Geometry check sheet. Reference: the model listing, model coordinates, mm. A direction names the side the tool comes from. Give positions to 0.01 mm unless a question says otherwise; leave off trailing zeros. Loops run counter-clockwise (first coordinate to the right, second up) from the corner with the lowest first, then second, coordinate; pieces in that order, holes last. Notation, with made-up numbers: (69, 62.5) -> (92, 62.5) arc R18 cw to (92, 83.5) -> close; hole circle Ø5 at (-32.5, 46). An arc over 180 degrees is marked (long way). Answer as a JSON object with one key per item and string values.
Autodesk Inventor part; units mm, degrees
ref_plane "YZ Plane" through (0, 0, 0) normal (1, 0, 0) x (0, 1, 0)
ref_plane "XZ Plane" through (0, 0, 0) normal (0, 1, 0) x (-1, 0, 0)
ref_plane "XY Plane" through (0, 0, 0) normal (0, 0, 1) x (1, 0, 0)
sketch "Sketch1" plane through (0, 0, 0) normal (0, 0, 1) x (1, 0, 0)
  line L0 (64, 0) -> (64, 36)
  line L1 (64, 36) -> (0, 36)
  line L2 (0, 36) -> (0, 0)
  line L3 (40, 0) -> (40, -9)
  line L4 (40, -9) -> (24, -9)
  line L5 (24, -9) -> (24, 0)
  line L6 (0, 0) -> (24, 0)
  line L7 (40, 0) -> (64, 0)
  dimension "d0" = 64
  dimension "d1" = 36
  dimension "d2" = 16
  dimension "d3" = 9
  dimension "d4" = 24
extrude "Extrusion1" add sketch "Sketch1" along normal blind 32
sketch "Sketch2" plane through (0, 0, 32) normal (0, 0, 1) x (1, 0, 0)
  circle A0 centre (32, 20) radius 6
  line L0 (0, 36) -> (0, 0)
  line L1 (40, 0) -> (64, 0)
  arc A1 (45.5949, 28.4368) -> (18.4051, 28.4368) centre (32, 20) ccw
  line L2 (0, 8.4474) -> (4.331, 8.4474)
  line L3 (6.8801, 9.8655) -> (18.4051, 28.4368)
  line L4 (64, 0) -> (64, 36)
  line L5 (64, 8.4474) -> (59.669, 8.4474)
  line L6 (57.1199, 9.8655) -> (45.5949, 28.4368)
  arc A2 (4.331, 8.4474) -> (6.8801, 9.8655) centre (4.331, 11.4474) ccw
  arc A3 (57.1199, 9.8655) -> (59.669, 8.4474) centre (59.669, 11.4474) ccw
  line L7 (0, 8.4474) -> (0, 36)
  line L8 (64, 36) -> (0, 36)
  line L9 (0, 36) -> (64, 36)
  line L10 (64, 36) -> (64, 8.4474)
  point P0 (6, 8.4474)
  point P1 (58, 8.4474)
  point P2 (32, 36)
  dimension "d7" = 12
  dimension "d8" = 32
  dimension "d9" = 20
  dimension "d10" = 6
  dimension "d11" = 32
  dimension "d12" = 6
  dimension "d13" = 3
extrude "Extrusion2" cut sketch "Sketch2" against normal blind 22 contours L8 A1 L3 A2 L2 L0 | L8 L4 L5 A3 L6 A1
sketch "Sketch3" plane through (0, 0, 32) normal (0, 0, 1) x (1, 0, 0)
  circle A0 centre (32, 20) radius 8
  line L0 (0, 8.4474) -> (0, 36)
  line L1 (40, 0) -> (64, 0)
  point P0 (0, 0)
  dimension "d16" = 16
  dimension "d17" = 32
  dimension "d18" = 20
extrude "Extrusion3" cut sketch "Sketch3" against normal blind 24
sketch "Sketch4" plane through (0, 36, 0) normal (0, 1, 0) x (1, 0, 0)
  circle A0 centre (32, -20) radius 3
  line L0 (18.4051, -32) -> (45.5949, -32)
  line L1 (0, -32) -> (0, -10)
  point P0 (0, 0)
  dimension "d21" = 6
  dimension "d22" = 12
  dimension "d23" = 32
extrude "Extrusion4" cut sketch "Sketch4" against normal blind 16
sketch "Sketch5" plane through (0, 36, 0) normal (0, 1, 0) x (1, 0, 0)
  circle A0 centre (32, -20) radius 5
  line L0 (18.4051, -32) -> (45.5949, -32)
  line L1 (0, -32) -> (0, -10)
  point P0 (0, 0)
  dimension "d26" = 10
  dimension "d27" = 12
  dimension "d28" = 32
extrude "Extrusion5" cut sketch "Sketch5" against normal blind 4
sketch "Sketch6" plane through (24, -9, 0) normal (0, -1, 0) x (1, 0, 0)
  circle A0 centre (8, 24) radius 3
  circle A1 centre (8, 8) radius 3
  line L0 (0, 32) -> (16, 32)
  point P0 (-24, 0)
  dimension "d31" = 6
  dimension "d32" = 6
  dimension "d33" = 8
  dimension "d34" = 16
extrude "Extrusion6" cut sketch "Sketch6" against normal blind 16
properties part number "third"
1) Section check A-A on z = 30. Record the cut outline in (x, y).
Geometry check:
{"outline": "(0, 0) -> (24, 0) -> (24, -9) -> (40, -9) -> (40, 0) -> (64, 0) -> (64, 8.45) -> (59.67, 8.45) arc R3 cw to (57.12, 9.87) -> (45.59, 28.44) arc R16 ccw to (18.41, 28.44) -> (6.88, 9.87) arc R3 cw to (4.33, 8.45) -> (0, 8.45) -> close; hole circle Ø16 at (32, 20)"}
2) Section check C-C on y = -5. Record the cut outline in (x, z).
Geometry check:
{"outline": "(24, 0) -> (40, 0) -> (40, 32) -> (24, 32) -> close; hole circle Ø6 at (32, 8); hole circle Ø6 at (32, 24)"}
3) Tool access check on faces 5 (the face through (28, 34, 23)), 6 (the face through (55, 25, 10)), 7 (the face through (12, 0, 16)), 8 (the face through (2, 8.447, 21)). Record the directions out of +Z, -Z, +X, -X, +Y, -Y that give a thin tool (end or side, any length) a straight path to the whole face; none if there is none.
Geometry check:
{"face 5": "+Y", "face 6": "+Z, +X, +Y", "face 7": "+Z, -Z, -X, -Y", "face 8": "+Z, -X, +Y"}
4) Depth check by flat-ended pin: P1, Ø5, axis at x = 62.5, z = 25.5, coming from the +Y side; P2, Ø6, axis at x = 15.5, z = 27.5, coming from the +Y side; P3, Ø3, axis at x = 30.5, z = 19, coming from the +Y side. Enter the tip coordinate at first touch or a pass-through.
Geometry check:
{"P1": "stops at y = 8.45", "P2": "stops at y = 28.59", "P3": "stops at y = 32"}
5) Section check D-D on z = 20. Record the cut outline in (x, y).
Geometry check:
{"outline": "(0, 0) -> (24, 0) -> (24, -9) -> (40, -9) -> (40, 0) -> (64, 0) -> (64, 8.45) -> (59.67, 8.45) arc R3 cw to (57.12, 9.87) -> (45.59, 28.44) arc R16 ccw to (37, 35.2) -> (37, 32) -> (35, 32) -> (35, 27.42) arc R8 cw (long way) to (29, 27.42) -> (29, 32) -> (27, 32) -> (27, 35.2) arc R16 ccw to (18.41, 28.44) -> (6.88, 9.87) arc R3 cw to (4.33, 8.45) -> (0, 8.45) -> close"}
6) Material ranges on line 1 along Z through (x, y) = (32, -2); line 2 along Y through (x, z) = (32, 23.75); line 3 along Z through (x, y) = (34, 6), recorded low to high. Write a range as from..to.
Geometry check:
{"line 1": "z = 0..5, 11..21, 27..32", "line 2": "y = 7..12, 28..32", "line 3": "z = 0..5.76, 10.24..21.76, 26.24..32"}
7) Draft check along X on faces 1 (the face through (64, 14, 9)), 2 (the face through (30.27, 12.19, 20.17)), 3 (the face through (52, 0, 16)), 4 (the face through (32, 7, 24)). Enter one of: pulls with the +X half, pulls with the -X half, needs draft (parallel to the pull), parting line crosses it, or undercut.
Geometry check:
{"face 1": "pulls with the +X half", "face 2": "undercut", "face 3": "needs draft", "face 4": "undercut"}
